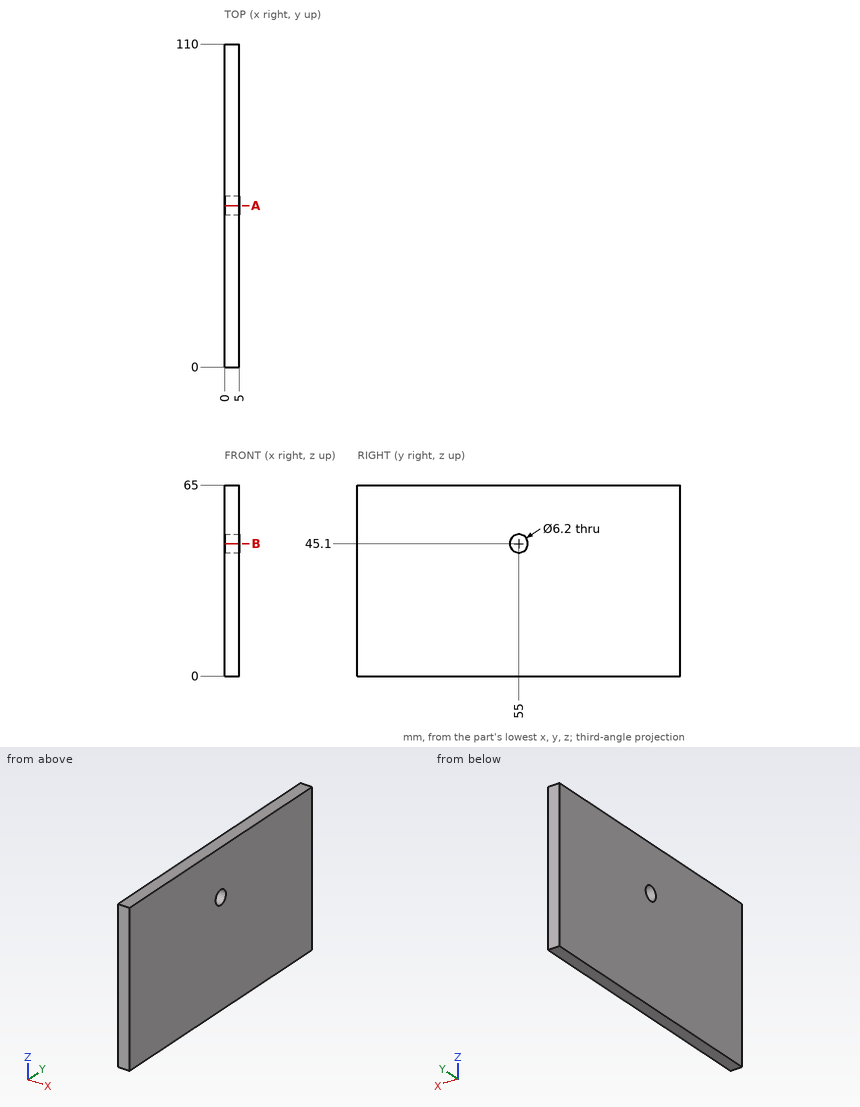
For this review, use the dimensioned drawing (mm, ordinates from the lowest corner) and the shaded views. Coordinates: 2 decimals unless noted, no trailing zeros. Loops run counter-clockwise (first coordinate to the right, second up) from the corner with the lowest first, then second, coordinate; pieces in that order, holes last. Notation, with made-up numbers: (-9, 82) -> (47, 82) arc R11 cw to (47, 91) -> close; hole circle Ø10 at (-20, -35). An arc over 180 degrees is marked (long way). Use a Markdown table: item, result. Add a question column.
1. To check wall thickness, follow line 1 (Z direction, x = 1.55, y = 55); line 2 (Y direction, x = 3.3, z = 44.5). State the ranges of each line that lie inside material, in increasing order.
2. Add section A-A on y = 55. Write out the cut boundary in (x, z).
3. Add section B-B on z = 45.1. Write out the cut boundary in (x, y), plus the area to 3 significant figures.
Returned:
| question | item | result |
|---|---|---|
| 1 | line 1 | z = 0 to 42, 48.2 to 65 |
| 1 | line 2 | y = 0 to 51.96, 58.04 to 110 |
| 2 | outline | (0, 0) -> (5, 0) -> (5, 42) -> (0, 42) -> close; (0, 48.2) -> (5, 48.2) -> (5, 65) -> (0, 65) -> close |
| 3 | outline | (0, 0) -> (5, 0) -> (5, 51.9) -> (0, 51.9) -> close; (0, 58.1) -> (5, 58.1) -> (5, 110) -> (0, 110) -> close |
| 3 | area | 519 mm² |
